Could you check a few things on this drawing? It's one solid part, dimensions in mm from its lowest x, y, z. A direction names the side the tool comes from. Give positions to 0.01 mm unless a question says otherwise; leave off trailing zeros. Write each loop counter-clockwise with the first axis right and the second up, starting at its lowest first coordinate (ties: lowest second). Pieces come first, ordered by that corner, then holes. Notation, with made-up numbers: M 69,46.25 L 87,46.25 A12 ccw 87,69.25 Z; hole C 3.5,-19 d7. An arc over 180 degrees is marked long. Answer as CSV lines item,"result". Start each with the question number.
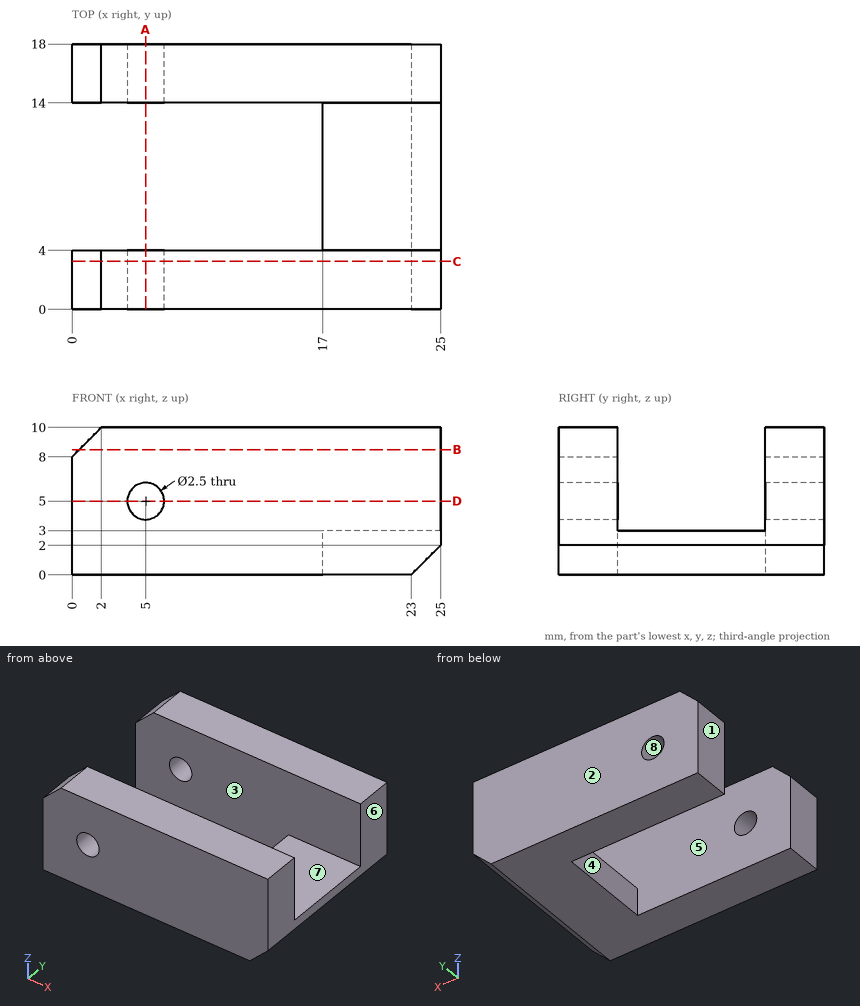
1) I want a section at B-B, the plane z = 8.5. Please give me the cut outline in (x, y), then the cut area to 3 significant figures.
2) Thinking about a two-plate mould opening in Y: for the marked faces 1, 2 and 3, which applies, released by +Y, released by -Y, zero draft, split by the parting line, or undercut?
3) I want a section at A-A, the plane x = 5. Please give me the cut outline in (y, z), then the cut area to 3 significant figures.
4) I want a section at D-D, the plane z = 5. Please give me the cut outline in (x, y), then the cut area to 3 significant figures.
5) On a 3-axis mill with a long thin cutter (end or side, diameter ignored), from which of +Z, -Z, +X, -X, +Y, -Y can I reach the whole of each face in a straight line? I mean the marked faces 4, 5, 6, 7 and 8. Say none if no direction works.
6) I need wall thicknesses on L1, parallel to Y at x = 7.5, z = 0.5; L2, parallel to Z at x = 5, y = 15.85; L3, parallel to Z at x = 20.5, y = 4.75. Which ranges of each line are inside material? Lowest first, please. Write a range as from..to.
7) I'm going to push flat-ended pins straight in: P1, Ø6.5, axis at x = 22, y = 8, coming from the +Z side; P2, Ø1.5, axis at y = 10.5, z = 2, coming from the -X side. Where does each tip first touch, or does it pass through?
8) I want a section at C-C, the plane y = 3.25. Please give me the cut outline in (x, z).
Values found:
1,outline,"M 0.5,0 L 25,0 L 25,4 L 0.5,4 Z; M 0.5,14 L 25,14 L 25,18 L 0.5,18 Z"
1,area,"196 mm²"
2,face 1,"zero draft"
2,face 2,"released by +Y"
2,face 3,"undercut"
3,outline,"M 0,0 L 4,0 L 4,3.75 L 0,3.75 Z; M 0,6.25 L 4,6.25 L 4,10 L 0,10 Z; M 14,0 L 18,0 L 18,3.75 L 14,3.75 Z; M 14,6.25 L 18,6.25 L 18,10 L 14,10 Z"
3,area,"60.0 mm²"
4,outline,"M 0,0 L 3.75,0 L 3.75,4 L 0,4 Z; M 0,14 L 3.75,14 L 3.75,18 L 0,18 Z; M 6.25,0 L 25,0 L 25,4 L 6.25,4 Z; M 6.25,14 L 25,14 L 25,18 L 6.25,18 Z"
4,area,"180 mm²"
5,face 4,"+Z, -Z, -X"
5,face 5,"+Z, -X"
5,face 6,"+Z, -Z, +X, +Y, -Y"
5,face 7,"+Z, +X, -X"
5,face 8,"+Y, -Y"
6,L1,"y = 0..4, 14..18"
6,L2,"z = 0..3.75, 6.25..10"
6,L3,"z = 0..3"
7,P1,"stops at z = 3"
7,P2,"stops at x = 17"
8,outline,"M 0,0 L 23,0 L 25,2 L 25,10 L 2,10 L 0,8 Z; hole C 5,5 d2.5"
